For this review, take the finished solid that the model builds, in its own axes (mm). A direction names the side the tool comes from. Round coordinates to 2 decimals unless told otherwise and drop trailing zeros. Loops run counter-clockwise (first coordinate to the right, second up) from the corner with the lowest first, then second, coordinate; pieces in that order, holes last. Notation, with made-up numbers: (18, 39.5) -> (68, 39.5) arc R36 cw to (68, 77.5) -> close; hole circle Ø2 at (-14, -18.75). An arc over 180 degrees is marked (long way). Write each question's results on one line, items separated by ' | '.
```python
from build123d import *

# Parameters (mm, degrees)
SKETCH2_R           = 12.7
SKETCH3_W           = 50.8
SKETCH3_H           = 50.8
BOSS_EXTRUDE1_DEPTH = 50.8
SKETCH4_R           = 12.7
BOSS_EXTRUDE2_DEPTH = 1528.8
SKETCH5_R           = 12.7
BOSS_EXTRUDE3_DEPTH = 1528.8


with BuildPart() as part:
    # Sweep1: sweep along a path in Sketch1
    with BuildLine(Plane.XY) as sweep1_path:
        Line((0, 0), (0, 203.2))
        ThreePointArc((0, 203.2), (37.197438789, 293.002561211), (127, 330.2))
        Line((127, 330.2), (1397, 330.2))
        ThreePointArc((1397, 330.2), (1486.802561211, 293.002561211), (1524, 203.2))
        Line((1524, 203.2), (1524, 0))
    # Sketch2 → Sweep1 (sweep)
    with BuildSketch(Plane(origin=(0, 0, 0), x_dir=(1, 0, 0), z_dir=(0, 1, 0))):
        Circle(SKETCH2_R)
    sweep(path=sweep1_path.line)

    # Sketch3 → Boss-Extrude1 (add)
    with BuildSketch(Plane.XZ):
        Rectangle(SKETCH3_W, SKETCH3_H)
        with Locations((1524, 0)):
            Rectangle(SKETCH3_W, SKETCH3_H)
    extrude(amount=BOSS_EXTRUDE1_DEPTH)

    # Sketch4 → Boss-Extrude2 (add)
    with BuildSketch(Plane(origin=(0, 0, 0), x_dir=(0, 0, -1), z_dir=(1, 0, 0))):
        with Locations((0, 203.2)):
            Circle(SKETCH4_R)
    extrude(amount=BOSS_EXTRUDE2_DEPTH)

    # Sketch5 → Boss-Extrude3 (add)
    with BuildSketch(Plane(origin=(0, 0, 0), x_dir=(0, 0, -1), z_dir=(1, 0, 0))):
        with Locations((0, 82.09908093)):
            Circle(SKETCH5_R)
    extrude(amount=BOSS_EXTRUDE3_DEPTH)


solid = part.part
```
1. Consider section A-A (z = 0). State the section outline as (x, y) points.
Values found:
outline: (-25.4, -50.8) -> (25.4, -50.8) -> (25.4, 0) -> (12.7, 0) -> (12.7, 69.4) -> (1511.3, 69.4) -> (1511.3, 0) -> (1498.6, 0) -> (1498.6, -50.8) -> (1549.4, -50.8) -> (1549.4, 0) -> (1536.7, 0) -> (1536.7, 203.2) arc R139.7 ccw to (1397, 342.9) -> (127, 342.9) arc R139.7 ccw to (-12.7, 203.2) -> (-12.7, 0) -> (-25.4, 0) -> close; hole (12.7, 94.8) -> (1511.3, 94.8) -> (1511.3, 190.5) -> (12.7, 190.5) -> close; hole (13.41, 215.9) -> (1510.59, 215.9) arc R114.3 ccw to (1397, 317.5) -> (127, 317.5) arc R114.3 ccw to start
2. Consider section B-B (y = 29.5). State the section outline as (x, z) points.
Values found:
outline: circle Ø25.4 at (0, 0); circle Ø25.4 at (1524, 0)
3. Draft analysis for pull direction X (two halves, no side actions). For faces 1 (the face through (0, -50.8, 0)), 2 (the face through (1549.4, -25, 0)), 3 (the face through (25.4, -25, 0)), state which applies: released by +X, released by -X, zero draft, split by the parting line, or undercut.
Values found:
face 1: zero draft | face 2: released by +X | face 3: undercut
4. Tool access review of faces 4 (the face through (1518, 0, 12)), 5 (the face through (1498.6, -25, 0)), 6 (the face through (-25.4, -25, 0)): name each direction out of +Z, -Z, +X, -X, +Y, -Y from which nothing blocks a thin tool from reaching the whole face with its end or side.
Values found:
face 4: none | face 5: +Z, -Z, -Y | face 6: +Z, -Z, -X, +Y, -Y
5. For pin 1 (1 mm diameter, centred on y = 83.5, z = 12, fed in from +X); pin 2 (6 mm diameter, centred on y = 264, z = -0.5, fed in from +X); pin 3 (6 mm diameter, centred on x = 791.5, z = 8.5, fed in from +Y); pin 4 (4 mm diameter, centred on x = 1308, z = 0.5, fed in from +Y), all flat-tipped, find the tip position at first contact; note any pin that passes through.
Values found:
pin 1: stops at x = 1529.39 | pin 2: stops at x = 1524.18 | pin 3: stops at y = 341.65 | pin 4: stops at y = 342.9
6. To check wall thickness, follow probe 1 along Y at (x, z) = (1184.5, -3); probe 2 along Y at (x, z) = (1068, 8); probe 3 along X at (y, z) = (-34, 15). State the ranges of each line that lie inside material, in increasing order.
Values found:
probe 1: y = 69.76 to 94.44, 190.86 to 215.54, 317.86 to 342.54 | probe 2: y = 72.24 to 91.96, 193.34 to 213.06, 320.34 to 340.06 | probe 3: x = -25.4 to 25.4, 1498.6 to 1549.4
7. Consider section C-C (x = 428). State the section outline as (y, z) points, plus the area to 3 significant figures.
Values found:
outline: circle Ø25.4 at (82.1, 0); circle Ø25.4 at (203.2, 0); circle Ø25.4 at (330.2, 0) | area: 1,520 mm2
